```python
from build123d import *

# Parameters (mm, degrees)
SKETCH1_W           = 203.2
SKETCH1_H           = 139.7
BOSS_EXTRUDE1_DEPTH = 50.8
SKETCH2_W           = 165.1
SKETCH2_H           = 38.1
CUT_EXTRUDE1_DEPTH  = 181.05357536
SKETCH3_R           = 11.1125
CUT_EXTRUDE2_DEPTH  = 181.05357536
FILLET1_R           = 12.7
FILLET3_R           = 12.7
FILLET2_R           = 2.54


with BuildPart() as part:
    # Sketch1 → Boss-Extrude1 (new body)
    with BuildSketch(Plane(origin=(0, 0, 0), x_dir=(1, 0, 0), z_dir=(0, 1, 0))):
        Rectangle(SKETCH1_W, SKETCH1_H)
    extrude(amount=BOSS_EXTRUDE1_DEPTH)

    # Sketch2 → Cut-Extrude1 (cut, through all)
    with BuildSketch(Plane.XY.offset(69.85)):
        with Locations((19.05, 31.75)):
            Rectangle(SKETCH2_W, SKETCH2_H)
    extrude(amount=-CUT_EXTRUDE1_DEPTH, mode=Mode.SUBTRACT)

    # Sketch3 → Cut-Extrude2 (cut, through all)
    with BuildSketch(Plane.XY.offset(69.85)):
        with Locations((-82.55, 25.4)):
            Circle(SKETCH3_R)
    extrude(amount=-CUT_EXTRUDE2_DEPTH, mode=Mode.SUBTRACT)

    # Fillet1
    fillet1_edges = [part.edges().sort_by_distance(p)[0] for p in [
        (-101.6, 50.8, 0),
        (-63.5, 12.7, 0),
        (-63.5, 50.8, 0),
    ]]
    fillet(fillet1_edges, radius=FILLET1_R)

    # Fillet3
    fillet3_edges = [part.edges().sort_by_distance(p)[0] for p in [
        (101.6, 6.35, 69.85),
        (101.6, 6.35, -69.85),
    ]]
    fillet(fillet3_edges, radius=FILLET3_R)

    # Fillet2
    fillet2_edges = [part.edges().sort_by_distance(p)[0] for p in [
        (19.05, 12.7, 69.85),
        (19.05, 12.7, -69.85),
        (-63.5, 31.75, 69.85),
        (-63.5, 31.75, -69.85),
        (-82.55, 50.8, -69.85),
        (-82.55, 50.8, 69.85),
        (-101.6, 19.05, 69.85),
        (-67.219743879, 47.080256121, 69.85),
        (-97.880256121, 47.080256121, 69.85),
        (-101.6, 19.05, -69.85),
        (-67.219743879, 47.080256121, -69.85),
        (-97.880256121, 47.080256121, -69.85),
        (-59.780256121, 16.419743879, 69.85),
        (-59.780256121, 16.419743879, -69.85),
        (-6.35, 0, 69.85),
        (-101.6, 0, 0),
        (-6.35, 0, -69.85),
        (101.6, 0, 0),
        (97.880256121, 0, 66.130256121),
        (97.880256121, 0, -66.130256121),
        (101.6, 12.7, 0),
        (97.880256121, 12.7, 66.130256121),
        (97.880256121, 12.7, -66.130256121),
    ]]
    fillet(fillet2_edges, radius=FILLET2_R)


solid = part.part
```
The listing builds one solid part. Answer for the finished solid, in the listing's coordinates (mm). A direction names the side the tool comes from. Give positions to 0.01 mm unless a question says otherwise; leave off trailing zeros. Order: outer loops, then holes, each group sorted by start corner. A loop starts at its lowest first (then second) coordinate and runs counter-clockwise, first axis right, second up. Notation, with made-up numbers: (27, -25) - (50, -25) arc R18 ccw to (50, -19) - close; hole circle Ø7 at (50, 40.25). An arc over 180 degrees is marked (long way). Answer in a Markdown table with one row per item. Add a question column.
Q1. Find the intervals of material crossed by line 1 along Y through (x, z) = (-83, 22.5); line 2 along X through (y, z) = (25, 18); line 3 along Y through (x, z) = (18, -5), in increasing order. Write a range as [from, to].
Q2. The part is cut by section B-B (x = -82.55). Determine the outline of the cut face in (y, z), then the cut area to 3 significant figures.
Q3. Given P1, Ø6.5, axis at y = 32.5, z = 9.5, coming from the +X side; P2, Ø8, axis at y = 44.5, z = 8, coming from the -X side; P3, Ø6, axis at x = 77, z = 19, coming from the +Y side; P4, Ø20, axis at x = -82.55, y = 25.4, coming from the -Z side, each flat-ended and moving along its own axis, determine where each tip first touches the part or whether it passes through.
Q4. Which of the six approach directions +Z, -Z, +X, -X, +Y, -Y give full straight-line access (tool end or side, diameter ignored) to faces 1 (the cylindrical face through (-72.285, 21.144, 0.978)), 2 (the flat face through (23, 12.7, 1))?
Q5. The part is cut by section C-C (x = 28.5). Determine the outline of the cut face in (y, z), then the cut area to 3 significant figures.
Determined:
| question | item | result |
|---|---|---|
| 1 | line 1 | y = [0, 14.3], [36.5, 50.8] |
| 1 | line 2 | x = [-101.6, -93.66], [-71.44, -63.49] |
| 1 | line 3 | y = [0, 12.7] |
| 2 | outline | (0, -67.31) arc R2.54 ccw to (2.54, -69.85) - (14.29, -69.85) - (14.29, 69.85) - (2.54, 69.85) arc R2.54 ccw to (0, 67.31) - close; (36.51, -69.85) - (48.26, -69.85) arc R2.54 ccw to (50.8, -67.31) - (50.8, 67.31) arc R2.54 ccw to (48.26, 69.85) - (36.51, 69.85) - close |
| 2 | area | 3,990 mm² |
| 3 | P1 | stops at x = -63.5 |
| 3 | P2 | stops at x = -101.37 |
| 3 | P3 | stops at y = 12.7 |
| 3 | P4 | passes through |
| 4 | face 1 | +Z, -Z |
| 4 | face 2 | +Z, -Z, +X, +Y |
| 5 | outline | (0, -67.31) arc R2.54 ccw to (2.54, -69.85) - (10.16, -69.85) arc R2.54 ccw to (12.7, -67.31) - (12.7, 67.31) arc R2.54 ccw to (10.16, 69.85) - (2.54, 69.85) arc R2.54 ccw to (0, 67.31) - close |
| 5 | area | 1,770 mm² |
